Verification items for the finished model (mm, model axes). A direction names the side the tool comes from. Round coordinates to 2 decimals unless told otherwise and drop trailing zeros. Order: outer loops, then holes, each group sorted by start corner. A loop starts at its lowest first (then second) coordinate and runs counter-clockwise, first axis right, second up. Notation, with made-up numbers: M -7,58 L 45,58 A14 ccw 45,75 Z; hole C -1.5,56 d7. An arc over 180 degrees is marked long. Return JSON: item names as keys, results as strings. Group by question number.
from build123d import *

# Parameters (mm, degrees)
SKETCH1_W           = 56
SKETCH1_H           = 82.5
SKETCH1_R           = 1.55
BOSS_EXTRUDE1_DEPTH = 5
SKETCH2_W           = 56
SKETCH2_H           = 82.5
SKETCH2_W_2         = 45
SKETCH2_H_2         = 71.5
BOSS_EXTRUDE2_DEPTH = 11.75
SKETCH3_W           = 5.5
SKETCH3_H           = 32.5
SKETCH3_W_2         = 41
SKETCH3_H_2         = 5.5
CUT_EXTRUDE1_DEPTH  = 11.75
FILLET1_R           = 1
SKETCH5_R           = 2.8
CUT_EXTRUDE2_DEPTH  = 3.1
SKETCH6_W           = 14.5
SKETCH6_H           = 28.330895985
CUT_EXTRUDE4_DEPTH  = 52.221333446


with BuildPart() as part:
    # Sketch1 → Boss-Extrude1 (new body)
    with BuildSketch(Plane(origin=(0, 0, 0), x_dir=(1, 0, 0), z_dir=(0, 1, 0))):
        Rectangle(SKETCH1_W, SKETCH1_H)
        with Locations(Location((-11.6, 0, 0), (0, 0, 270))):
            Circle(SKETCH1_R, mode=Mode.SUBTRACT)
        with Locations(Location((0, -11.75, 0), (0, 0, 270))):
            Circle(SKETCH1_R, mode=Mode.SUBTRACT)
        with Locations(Location((11.6, -0.25, 0), (0, 0, 270))):
            Circle(SKETCH1_R, mode=Mode.SUBTRACT)
    extrude(amount=BOSS_EXTRUDE1_DEPTH)

    # Sketch2 → Boss-Extrude2 (add)
    with BuildSketch(Plane(origin=(0, 5, 0), x_dir=(1, 0, 0), z_dir=(0, 1, 0))):
        Rectangle(SKETCH2_W, SKETCH2_H)
        Rectangle(SKETCH2_W_2, SKETCH2_H_2, mode=Mode.SUBTRACT)
    extrude(amount=BOSS_EXTRUDE2_DEPTH)

    # Sketch3 → Cut-Extrude1 (cut)
    with BuildSketch(Plane(origin=(0, 16.75, 0), x_dir=(1, 0, 0), z_dir=(0, 1, 0))):
        with Locations((-25.25, 0)):
            Rectangle(SKETCH3_W, SKETCH3_H)
        with Locations((0, 38.5)):
            Rectangle(SKETCH3_W_2, SKETCH3_H_2)
        with Locations((0, -38.5)):
            Rectangle(SKETCH3_W_2, SKETCH3_H_2)
        with Locations((25.25, 0)):
            Rectangle(SKETCH3_W, SKETCH3_H)
    extrude(amount=-CUT_EXTRUDE1_DEPTH, mode=Mode.SUBTRACT)

    # Fillet1
    fillet1_edges = [part.edges().sort_by_distance(p)[0] for p in [
        (22.5, 5, 26),
        (21.5, 5, -35.75),
        (-22.5, 5, -26),
        (-21.5, 5, 35.75),
        (21.5, 5, 35.75),
        (-22.5, 5, 26),
        (-21.5, 5, -35.75),
        (22.5, 5, -26),
        (-25.25, 5, 16.25),
        (-25.25, 5, -16.25),
        (20.5, 5, -38.5),
        (-20.5, 5, -38.5),
        (20.5, 5, 38.5),
        (-20.5, 5, 38.5),
        (25.25, 5, 16.25),
        (25.25, 5, -16.25),
    ]]
    fillet(fillet1_edges, radius=FILLET1_R)

    # Sketch5 → Cut-Extrude2 (cut)
    with BuildSketch(Plane(origin=(0, 5, 0), x_dir=(1, 0, 0), z_dir=(0, 1, 0))):
        with Locations(Location((-11.6, 0, 0), (0, 0, 270))):
            Circle(SKETCH5_R)
        with Locations(Location((11.6, -0.25, 0), (0, 0, 270))):
            Circle(SKETCH5_R)
        with Locations(Location((0, -11.75, 0), (0, 0, 270))):
            Circle(SKETCH5_R)
    extrude(amount=-CUT_EXTRUDE2_DEPTH, mode=Mode.SUBTRACT)

    # Sketch6 → Cut-Extrude4 (cut, through all)
    with BuildSketch(Plane(origin=(0, 5, 0), x_dir=(1, 0, 0), z_dir=(0, 1, 0))):
        with Locations((-11.25, 18.165447993)):
            Rectangle(SKETCH6_W, SKETCH6_H)
        with Locations((11.25, 18.165447993)):
            Rectangle(SKETCH6_W, SKETCH6_H)
        with Locations((11.25, -18.165447993)):
            Rectangle(SKETCH6_W, SKETCH6_H)
        with Locations((-11.25, -18.165447993)):
            Rectangle(SKETCH6_W, SKETCH6_H)
    extrude(amount=-CUT_EXTRUDE4_DEPTH, mode=Mode.SUBTRACT)


solid = part.part
1. Cross-section at A-A (y = 12.25). Enter the section's corners in (x, z), plus the area to 3 significant figures.
2. Go/stop test with flat-tipped pins: pin 1 (1.9 mm diameter, centred on x = 11.6, z = 0.25, fed in from +Y); pin 2 (6 mm diameter, centred on x = -0.5, z = 11, fed in from +Y). Record where each tip stops, or that it passes through.
3. Cross-section at B-B (z = 11.75). Enter the section's corners in (x, y), plus the area to 3 significant figures.
4. Cross-section at D-D (z = -31.5). Enter the section's corners in (x, y), plus the area to 3 significant figures.
5. Access from +Z, -Z, +X, -X, +Y, -Y to the whole of each face (thin tool, end or side, straight path). Record for faces 1 (the face through (28, 4.5, 0.6)), 2 (the face through (18.5, 3, -18)), 3 (the face through (-20.5, 11, -38)), 4 (the face through (-13.304, 3.472, -2.222)).
6. Draft check along Z on faces 5 (the face through (-0.4, 4.5, 41.25)), 6 (the face through (-22.5, 11, -26)), 7 (the face through (-20.5, 11, 39)). Enter one of: +Z half, -Z half, draft (parallel to the pull), parting line (faces both ways), or undercut.
7. Thickness scan on line 1 along Z through (x, y) = (11.6, 0.7); line 2 along X through (y, z) = (1, 26); line 3 along Z through (x, y) = (-11.6, 1.35). Record the ranges inside material, lowest first. Write a range as from..to.
8. Cross-section at C-C (x = -11.6). Enter the section's corners in (y, z), plus the area to 3 significant figures.
Computed:
{
 "1": {"outline": "M -28,-41.25 L -20.5,-41.25 L -20.5,-35.75 L -22.5,-35.75 L -22.5,-16.25 L -28,-16.25 Z; M -28,16.25 L -22.5,16.25 L -22.5,35.75 L -20.5,35.75 L -20.5,41.25 L -28,41.25 Z; M 20.5,-41.25 L 28,-41.25 L 28,-16.25 L 22.5,-16.25 L 22.5,-35.75 L 20.5,-35.75 Z; M 20.5,35.75 L 22.5,35.75 L 22.5,16.25 L 28,16.25 L 28,41.25 L 20.5,41.25 Z", "area": "594 mm²"},
 "2": {"pin 1": "passes through", "pin 2": "stops at y = 5"},
 "3": {"outline": "M -28,0 L -18.5,0 L -18.5,5 L -28,5 Z; M -4,0 L -1.55,0 L -1.55,1.9 L -2.8,1.9 L -2.8,5 L -4,5 Z; M 1.55,0 L 4,0 L 4,5 L 2.8,5 L 2.8,1.9 L 1.55,1.9 Z; M 18.5,0 L 28,0 L 28,5 L 18.5,5 Z", "area": "112 mm²"},
 "4": {"outline": "M -28,0 L -18.5,0 L -18.5,5 L -21.5,5 A1 cw -22.5,6 L -22.5,16.75 L -28,16.75 Z; M -4,0 L 4,0 L 4,5 L -4,5 Z; M 18.5,0 L 28,0 L 28,16.75 L 22.5,16.75 L 22.5,6 A1 cw 21.5,5 L 18.5,5 Z", "area": "265 mm²"},
 "5": {"face 1": "+Z, -Z, +X, +Y, -Y", "face 2": "+Y, -Y", "face 3": "+Z, -Z, +Y", "face 4": "+Y"},
 "6": {"face 5": "+Z half", "face 6": "undercut", "face 7": "draft"},
 "7": {"line 1": "z = -41.25..-32.33, -4..-1.3, 1.8..4, 32.33..41.25", "line 2": "x = -28..-18.5, -4..4, 18.5..28", "line 3": "z = -41.25..-32.33, -4..-1.55, 1.55..4, 32.33..41.25"},
 "8": {"outline": "M 0,-41.25 L 5,-41.25 L 5,-32.33 L 0,-32.33 Z; M 0,-4 L 5,-4 L 5,-2.8 L 1.9,-2.8 L 1.9,-1.55 L 0,-1.55 Z; M 0,1.55 L 1.9,1.55 L 1.9,2.8 L 5,2.8 L 5,4 L 0,4 Z; M 0,32.33 L 5,32.33 L 5,41.25 L 0,41.25 Z", "area": "106 mm²"}
}
